from build123d import *

# Parameters (mm, degrees)
SKETCH1_R           = 32.5
BOSS_EXTRUDE1_DEPTH = 40
SKETCH2_R           = 3
CUT_EXTRUDE1_DEPTH  = 63


with BuildPart() as part:
    # Sketch1 → Boss-Extrude1 (new body)
    with BuildSketch(Plane.XY):
        Polygon((0, 0), (102, 0), (102, 62), (85, 62), (66, 81), (36, 81), (17, 62), (0, 62), align=None)
        with Locations((51, 40.5)):
            Circle(SKETCH1_R, mode=Mode.SUBTRACT)
    extrude(amount=BOSS_EXTRUDE1_DEPTH)

    # Sketch2 → Cut-Extrude1 (cut, through all)
    with BuildSketch(Plane(origin=(0, 62, 0), x_dir=(1, 0, 0), z_dir=(0, 1, 0))):
        with Locations((6, -5)):
            Circle(SKETCH2_R)
        with Locations((6, -35)):
            Circle(SKETCH2_R)
        with Locations((96, -5)):
            Circle(SKETCH2_R)
        with Locations((96, -35)):
            Circle(SKETCH2_R)
    extrude(amount=-CUT_EXTRUDE1_DEPTH, mode=Mode.SUBTRACT)


solid = part.part
The listing builds one solid part. Answer for the finished solid, in the listing's coordinates (mm). A direction names the side the tool comes from. Coordinates: 2 decimals unless noted, no trailing zeros. Order: outer loops, then holes, each group sorted by start corner. A loop starts at its lowest first (then second) coordinate and runs counter-clockwise, first axis right, second up. Notation, with made-up numbers: (78, 53.25) -> (126, 53.25) arc R21 cw to (126, 74.25) -> close; hole circle Ø4 at (70.5, 36). An arc over 180 degrees is marked (long way). Answer in a Markdown table with one row per item. Add a question column.
Item 1: Which of the six approach directions +Z, -Z, +X, -X, +Y, -Y give full straight-line access (tool end or side, diameter ignored) to faces 5 (the face through (93, 31, 5)), 6 (the face through (9, 62, 20)), 7 (the face through (94, 62, 20))?
Item 2: Determine the mould class of faces 1 (the face through (50, 0, 20)), 2 (the face through (0, 31, 20)), 3 (the face through (6, 31, 32)), 4 (the face through (102, 31, 20)) for opening direction X: +X half, -X half, draft (parallel to the pull), parting line (faces both ways), or undercut.
Item 3: Find section A-A (z = 5). Write down the section's boundary in (x, y).
Item 4: Find section D-D (z = 26). Write down the section's boundary in (x, y), then the cut area to 3 significant figures.
Item 5: Each of these flat-tipped pins is pushed along its axis until it touches: P1, Ø1.5, axis at x = 68.5, z = 9, coming from the +Y side; P2, Ø18.5, axis at x = 10.5, z = 24, coming from the +Y side; P3, Ø8, axis at x = 6, z = 5, coming from the +Y side; P4, Ø3.5, axis at x = 96, z = 35, coming from the -Y side (3 decimals). Where does it stop, or does it pass through?
Item 6: Find the intervals of material crossed by L1, parallel to X at y = 41, z = 35; L2, parallel to Z at x = 96, y = 19; L3, parallel to Y at x = 50, z = 30.5, in increasing order. Write a range as from..to.
Item 7: Find section C-C (y = 35). Write down the section's boundary in (x, z), then the cut area to 3 significant figures.
Item 8: Find section B-B (x = 6). Write down the section's boundary in (y, z).
Result set:
| question | item | result |
|---|---|---|
| 1 | face 5 | +Y, -Y |
| 1 | face 6 | +Z, -Z, -X, +Y |
| 1 | face 7 | +Z, -Z, +X, +Y |
| 2 | face 1 | draft |
| 2 | face 2 | -X half |
| 2 | face 3 | undercut |
| 2 | face 4 | +X half |
| 3 | outline | (0, 0) -> (3, 0) -> (3, 62) -> (0, 62) -> close; (9, 0) -> (93, 0) -> (93, 62) -> (85, 62) -> (66, 81) -> (36, 81) -> (17, 62) -> (9, 62) -> close; (99, 0) -> (102, 0) -> (102, 62) -> (99, 62) -> close; hole circle Ø65 at (51, 40.5) |
| 4 | outline | (0, 0) -> (102, 0) -> (102, 62) -> (85, 62) -> (66, 81) -> (36, 81) -> (17, 62) -> (0, 62) -> close; hole circle Ø65 at (51, 40.5) |
| 4 | area | 3,940 mm² |
| 5 | P1 | stops at y = 79.25 |
| 5 | P2 | stops at y = 64.75 |
| 5 | P3 | stops at y = 62 |
| 5 | P4 | passes through |
| 6 | L1 | x = 0..3, 9..18.5, 83.5..93, 99..102 |
| 6 | L2 | z = 0..2, 8..32, 38..40 |
| 6 | L3 | y = 0..8.02, 72.98..81 |
| 7 | outline | (0, 0) -> (18.97, 0) -> (18.97, 40) -> (0, 40) -> close; (83.03, 0) -> (102, 0) -> (102, 40) -> (83.03, 40) -> close; hole circle Ø6 at (6, 5); hole circle Ø6 at (6, 35); hole circle Ø6 at (96, 5); hole circle Ø6 at (96, 35) |
| 7 | area | 1,400 mm² |
| 8 | outline | (0, 0) -> (62, 0) -> (62, 2) -> (0, 2) -> close; (0, 8) -> (62, 8) -> (62, 32) -> (0, 32) -> close; (0, 38) -> (62, 38) -> (62, 40) -> (0, 40) -> close |
